Can you work these out from the model? Positions are in its coordinate system, mm. Face numbers are marked on the shaded views. A direction names the side the tool comes from. Give positions to 0.01 mm unless a question says otherwise; leave off trailing zeros. Loops run counter-clockwise (first coordinate to the right, second up) from the corner with the lowest first, then second, coordinate; pieces in that order, holes last. Notation, with made-up numbers: (-23, -38) - (16, -38) arc R33 ccw to (16, -3) - close; hole circle Ø8 at (-39, 5). An arc over 180 degrees is marked (long way). Answer as a JSON object with one key per item and string values.
```python
from build123d import *

# Parameters (mm, degrees)
SKETCH1_W           = 150
SKETCH1_H           = 64
BOSS_EXTRUDE1_DEPTH = 94
SKETCH2_W           = 64
SKETCH2_H           = 6
CUT_EXTRUDE1_DEPTH  = 2
CUT_EXTRUDE2_DEPTH  = 2
SKETCH4_W           = 130
SKETCH4_H           = 6
CUT_EXTRUDE3_DEPTH  = 2
SKETCH5_W           = 126
SKETCH5_H           = 56
CUT_EXTRUDE4_DEPTH  = 0.5
SKETCH6_W           = 14
SKETCH6_H           = 14
CUT_EXTRUDE5_DEPTH  = 1
SKETCH7_W           = 1
SKETCH7_H           = 6
BOSS_EXTRUDE2_DEPTH = 6
SKETCH8_W           = 4
SKETCH8_H           = 1
BOSS_EXTRUDE3_DEPTH = 8
SKETCH9_R           = 1
CUT_EXTRUDE6_DEPTH  = 1
SKETCH13_W          = 64
SKETCH13_H          = 80
CUT_EXTRUDE7_DEPTH  = 0.5
SKETCH14_W          = 149.5
SKETCH14_H          = 80
CUT_EXTRUDE8_DEPTH  = 0.5
SKETCH15_W          = 149.5
SKETCH15_H          = 80
CUT_EXTRUDE9_DEPTH  = 0.5
SKETCH16_W          = 63
SKETCH16_H          = 80
CUT_EXTRUDE10_DEPTH = 0.5
SKETCH17_R          = 3
CUT_EXTRUDE11_DEPTH = 1
SKETCH18_W          = 1
SKETCH18_H          = 5
BOSS_EXTRUDE4_DEPTH = 0.5
FILLET4_R           = 1
FILLET5_R           = 1


with BuildPart() as part:
    # Sketch1 → Boss-Extrude1 (new body)
    with BuildSketch(Plane(origin=(0, 0, 0), x_dir=(1, 0, 0), z_dir=(0, 1, 0))):
        Rectangle(SKETCH1_W, SKETCH1_H)
    extrude(amount=BOSS_EXTRUDE1_DEPTH)

    # Sketch2 → Cut-Extrude1 (cut)
    with BuildSketch(Plane(origin=(75, 0, 0), x_dir=(0, 0, -1), z_dir=(1, 0, 0))):
        with Locations((0, 91)):
            Rectangle(SKETCH2_W, SKETCH2_H)
    extrude(amount=-CUT_EXTRUDE1_DEPTH, mode=Mode.SUBTRACT)

    # Sketch3 → Cut-Extrude2 (cut)
    with BuildSketch(Plane(origin=(0, 0, -32), x_dir=(-1, 0, 0), z_dir=(0, 0, -1))):
        Polygon((-73, 88), (55, 88), (55, 94), (-73, 94), (-75, 94), (-75, 88), align=None)
    extrude(amount=-CUT_EXTRUDE2_DEPTH, mode=Mode.SUBTRACT)

    # Sketch4 → Cut-Extrude3 (cut)
    with BuildSketch(Plane.XY.offset(32)):
        with Locations((10, 91)):
            Rectangle(SKETCH4_W, SKETCH4_H)
    extrude(amount=-CUT_EXTRUDE3_DEPTH, mode=Mode.SUBTRACT)

    # Sketch5 → Cut-Extrude4 (cut)
    with BuildSketch(Plane(origin=(0, 94, 0), x_dir=(1, 0, 0), z_dir=(0, 1, 0))):
        with Locations((8, 0)):
            Rectangle(SKETCH5_W, SKETCH5_H)
    extrude(amount=-CUT_EXTRUDE4_DEPTH, mode=Mode.SUBTRACT)

    # Sketch6 → Cut-Extrude5 (cut)
    with BuildSketch(Plane(origin=(0, 94, 0), x_dir=(1, 0, 0), z_dir=(0, 1, 0))):
        with Locations((-65, -22)):
            Rectangle(SKETCH6_W, SKETCH6_H)
        with Locations((-65, 22)):
            Rectangle(SKETCH6_W, SKETCH6_H)
    extrude(amount=-CUT_EXTRUDE5_DEPTH, mode=Mode.SUBTRACT)

    # Sketch7 → Boss-Extrude2 (add)
    with BuildSketch(Plane(origin=(0, 93, 0), x_dir=(1, 0, 0), z_dir=(0, 1, 0))):
        with Locations((-60.5, 22)):
            Rectangle(SKETCH7_W, SKETCH7_H)
        with Locations((-60.5, -22)):
            Rectangle(SKETCH7_W, SKETCH7_H)
    extrude(amount=BOSS_EXTRUDE2_DEPTH)

    # Sketch8 → Boss-Extrude3 (add)
    with BuildSketch(Plane(origin=(-60, 0, 0), x_dir=(0, 0, -1), z_dir=(1, 0, 0))):
        with Locations((-22, 98.5)):
            Rectangle(SKETCH8_W, SKETCH8_H)
        with Locations((22, 98.5)):
            Rectangle(SKETCH8_W, SKETCH8_H)
    extrude(amount=BOSS_EXTRUDE3_DEPTH)

    # Sketch9 → Cut-Extrude6 (cut)
    with BuildSketch(Plane(origin=(0, 99, 0), x_dir=(1, 0, 0), z_dir=(0, 1, 0))):
        with Locations((-55, 22)):
            Circle(SKETCH9_R)
        with Locations((-55, -22)):
            Circle(SKETCH9_R)
    extrude(amount=-CUT_EXTRUDE6_DEPTH, mode=Mode.SUBTRACT)

    # Sketch13 → Cut-Extrude7 (cut)
    with BuildSketch(Plane(origin=(75, 0, 0), x_dir=(0, 0, -1), z_dir=(1, 0, 0))):
        with Locations((0, 40)):
            Rectangle(SKETCH13_W, SKETCH13_H)
    extrude(amount=-CUT_EXTRUDE7_DEPTH, mode=Mode.SUBTRACT)

    # Sketch14 → Cut-Extrude8 (cut)
    with BuildSketch(Plane.XY.offset(32)):
        with Locations((-0.25, 40)):
            Rectangle(SKETCH14_W, SKETCH14_H)
    extrude(amount=-CUT_EXTRUDE8_DEPTH, mode=Mode.SUBTRACT)

    # Sketch15 → Cut-Extrude9 (cut)
    with BuildSketch(Plane(origin=(0, 0, -32), x_dir=(-1, 0, 0), z_dir=(0, 0, -1))):
        with Locations((0.25, 40)):
            Rectangle(SKETCH15_W, SKETCH15_H)
    extrude(amount=-CUT_EXTRUDE9_DEPTH, mode=Mode.SUBTRACT)

    # Sketch16 → Cut-Extrude10 (cut)
    with BuildSketch(Plane.ZY.offset(75)):
        with Locations((0, 40)):
            Rectangle(SKETCH16_W, SKETCH16_H)
    extrude(amount=-CUT_EXTRUDE10_DEPTH, mode=Mode.SUBTRACT)

    # Sketch17 → Cut-Extrude11 (cut)
    with BuildSketch(Plane(origin=(0, 94, 0), x_dir=(1, 0, 0), z_dir=(0, 1, 0))):
        with Locations((-65, 9.5)):
            Circle(SKETCH17_R)
        with Locations((-65, -9.5)):
            Circle(SKETCH17_R)
    extrude(amount=-CUT_EXTRUDE11_DEPTH, mode=Mode.SUBTRACT)

    # Sketch18 → Boss-Extrude4 (add)
    with BuildSketch(Plane(origin=(0, 93, 0), x_dir=(1, 0, 0), z_dir=(0, 1, 0))):
        Polygon((-65.5, 12), (-64.5, 12), (-64.5, 10), (-62.5, 10), (-62.5, 9), (-64.5, 9), (-64.5, 7), (-65.5, 7), (-65.5, 9), (-67.5, 9), (-67.5, 10), (-65.5, 10), align=None)
        with Locations((-65, -9.5)):
            Rectangle(SKETCH18_W, SKETCH18_H)
    extrude(amount=BOSS_EXTRUDE4_DEPTH)

    # Fillet4
    fillet4_edges = [part.edges().sort_by_distance(p)[0] for p in [
        (74.5, 0, 0),
        (74.5, 40, 31.5),
        (74.5, 40, -31.5),
        (0, 0, -31.5),
        (0, 0, 31.5),
        (-74.5, 40, 31.5),
        (-74.5, 0, 0),
        (-74.5, 40, -31.5),
    ]]
    fillet(fillet4_edges, radius=FILLET4_R)

    # Fillet5
    fillet5_edges = [part.edges().sort_by_distance(p)[0] for p in [
        (-75, 94, 0),
        (-65, 94, 32),
        (75, 84, 32),
        (75, 84, -32),
        (10, 88, -32),
        (10, 88, 32),
        (75, 88, 0),
        (73, 94, 0),
        (73, 91, -30),
        (-65, 94, -32),
        (9, 94, -30),
        (-55, 91, -32),
        (73, 91, 30),
        (9, 94, 30),
        (-55, 91, 32),
        (-75, 87, 32),
        (-75, 87, -32),
    ]]
    fillet(fillet5_edges, radius=FILLET5_R)


solid = part.part
```
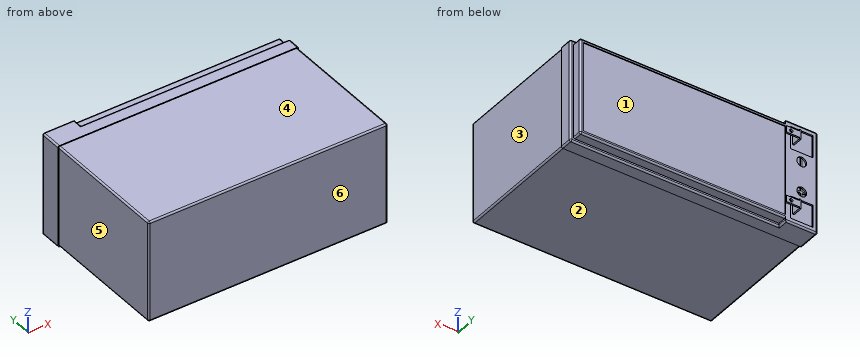
1) Imagine slicing it at A-A on y = 35. Write out the boundary of the cut face in (x, z).
Check sheet entries:
{"outline": "(-74.5, -30.5) arc R1 ccw to (-73.5, -31.5) - (73.5, -31.5) arc R1 ccw to (74.5, -30.5) - (74.5, 30.5) arc R1 ccw to (73.5, 31.5) - (-73.5, 31.5) arc R1 ccw to (-74.5, 30.5) - close"}
2) I'm going to push flat-ended pins straight in: P1, Ø5, axis at x = -22.5, y = 34, coming from the -Z side; P2, Ø0.6, axis at x = -67, y = 93.5, coming from the +Z side; P3, Ø0.5, axis at y = 98.5, z = 21.5, coming from the +X side. Where does each tip first touch, or does it pass through?
Check sheet entries:
{"P1": "z = -31.5", "P2": "z = 31.98", "P3": "x = -52"}
3) Imagine slicing it at B-B on x = 56. Write out the boundary of the cut face in (y, z), and give its area (3 significant figures).
Check sheet entries:
{"outline": "(0, -30.5) arc R1 ccw to (1, -31.5) - (80, -31.5) - (80, -32) - (87, -32) arc R1 ccw to (88, -31) - (88, -30) - (93, -30) arc R1 ccw to (94, -29) - (94, -28) - (93.5, -28) - (93.5, 28) - (94, 28) - (94, 29) arc R1 ccw to (93, 30) - (88, 30) - (88, 31) arc R1 ccw to (87, 32) - (80, 32) - (80, 31.5) - (1, 31.5) arc R1 ccw to (0, 30.5) - close", "area": "5,880 mm2"}
4) If we mould it in two halves opening along Z, with no side actions, what happens to the marked faces 1, 2 and 3? For each: released by +Z, released by -Z, zero draft, split by the parting line, or undercut.
Check sheet entries:
{"face 1": "undercut", "face 2": "released by -Z", "face 3": "zero draft"}
5) Which directions (+Z, -Z, +X, -X, +Y, -Y) give clear straight access to the entire face, cutting with the end or side of a thin tool? Please do the marked faces 4, 5 and 6.
Check sheet entries:
{"face 4": "+Z, +X, -X, -Y", "face 5": "+Z, -Z, -X, -Y", "face 6": "+Z, -Z, +X, -X, -Y"}
6) I need wall thicknesses on L1, parallel to Z at x = -55, y = 98.8; L2, parallel to X at y = 93.2, z = 9.5; L3, parallel to X at y = 98.75, z = 22. Which ranges of each line are inside material? Lowest first, please.
Check sheet entries:
{"L1": "-24 to -23, -21 to -20, 20 to 21, 23 to 24", "L2": "-74.98 to -68, -65.5 to -64.5, -62 to 72.98", "L3": "-61 to -56, -54 to -52"}
